For this review, use the dimensioned drawing (mm, ordinates from the lowest corner) and the shaded views. Coordinates: 2 decimals unless noted, no trailing zeros. Write each loop counter-clockwise with the first axis right and the second up, starting at its lowest first coordinate (ties: lowest second). Pieces come first, ordered by that corner, then holes. Notation, with made-up numbers: (39, 8) -> (52, 8) arc R21 cw to (52, 22) -> close; hole circle Ø1 at (75, 42.25). An arc over 180 degrees is marked (long way). Return JSON: item names as keys, results as strings. Group by question number.
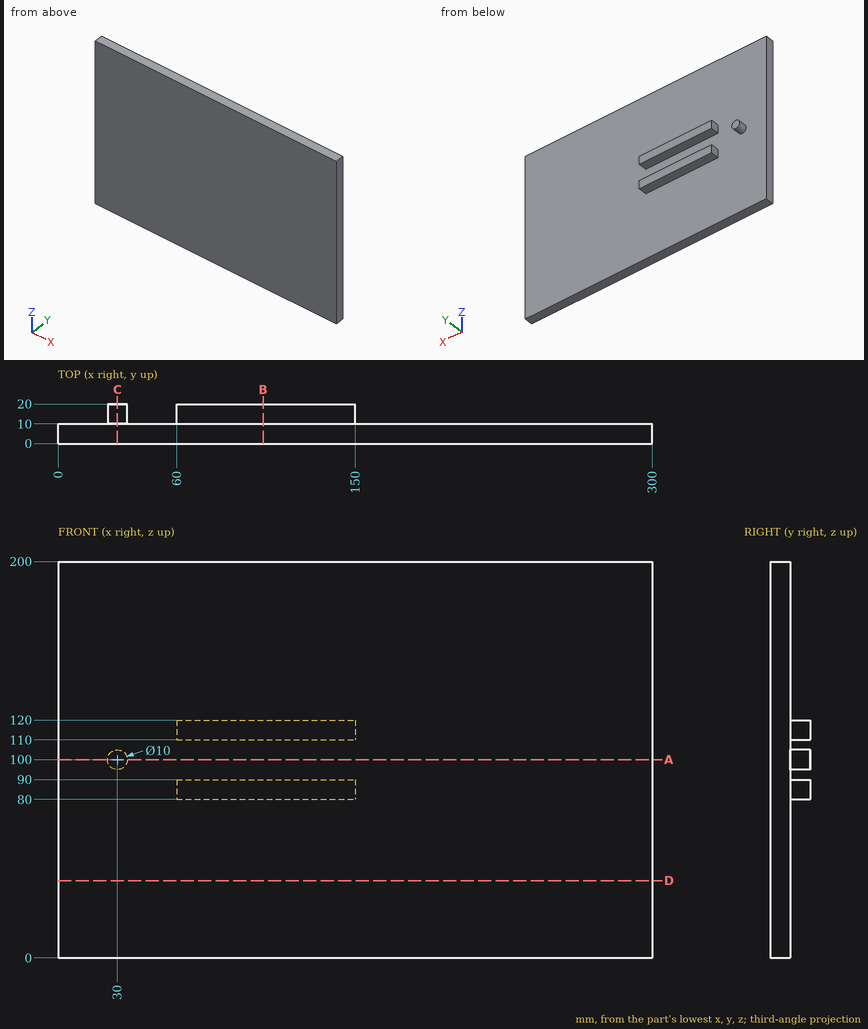
Q1. We need section A-A on z = 100. Write out the cut boundary in (x, y), plus the area to 3 significant figures.
Q2. For P1, Ø5, axis at x = 93, y = 13.5, coming from the +Z side; P2, Ø6, axis at y = 14, z = 114.5, coming from the -X side; P3, Ø3, axis at x = 113.5, y = 17.5, coming from the -Z side, all flat-tipped, find the tip position at first contact; note any pin that passes through.
Q3. We need section D-D on z = 39. Write out the cut boundary in (x, y), plus the area to 3 significant figures.
Q4. Wall thickness on L1, parallel to Z at x = 135.5, y = 10.25; L2, parallel to Y at x = 238, z = 83; L3, parallel to X at y = 18, z = 84.5: over which ranges is each line inside the solid? List them lowest first.
Q5. We need section B-B on x = 103.5. Write out the cut boundary in (y, z).
Q6. We need section C-C on x = 30. Write out the cut boundary in (y, z).
Findings below:
{
 "1": {"outline": "(0, 0) -> (300, 0) -> (300, 10) -> (35, 10) -> (35, 20) -> (25, 20) -> (25, 10) -> (0, 10) -> close", "area": "3,100 mm^2"},
 "2": {"P1": "stops at z = 120", "P2": "stops at x = 60", "P3": "stops at z = 80"},
 "3": {"outline": "(0, 0) -> (300, 0) -> (300, 10) -> (0, 10) -> close", "area": "3,000 mm^2"},
 "4": {"L1": "z = 80 to 90, 110 to 120", "L2": "y = 0 to 10", "L3": "x = 60 to 150"},
 "5": {"outline": "(0, 0) -> (10, 0) -> (10, 80) -> (20, 80) -> (20, 90) -> (10, 90) -> (10, 110) -> (20, 110) -> (20, 120) -> (10, 120) -> (10, 200) -> (0, 200) -> close"},
 "6": {"outline": "(0, 0) -> (10, 0) -> (10, 95) -> (20, 95) -> (20, 105) -> (10, 105) -> (10, 200) -> (0, 200) -> close"}
}
